```python
from build123d import *

# Parameters (mm, degrees)
F0_R     = 1.5
F1_DEPTH = 2.5


with BuildPart() as f1:
    # F0 (on Top) → F1 (new body)
    with BuildSketch(Plane.XY):
        Polygon((-24.927709, 2.481071), (7.530662, -30.014294), (11.431097, -31.130232), (23.566268, -40.223594), (34.787399, -29.015238), (46.00853, -17.806882), (36.928996, -5.66136), (35.817502, -1.759657), (3.359131, 30.735708), (-0.541304, 31.851646), (-12.676475, 40.945009), (-23.897606, 29.736653), (-35.118737, 18.528296), (-26.039203, 6.382775), align=None)
        with Locations((5.432613, -21.206046)):
            Circle(F0_R, mode=Mode.SUBTRACT)
        with Locations((23.566268, -33.655995)):
            Circle(F0_R, mode=Mode.SUBTRACT)
        with Locations((39.440935, -17.799401)):
            Circle(F0_R, mode=Mode.SUBTRACT)
        with Locations((27.01165, 0.348424)):
            Circle(F0_R, mode=Mode.SUBTRACT)
        with Locations((-16.121857, 0.372991)):
            Circle(F0_R, mode=Mode.SUBTRACT)
        with Locations((-28.551142, 18.520815)):
            Circle(F0_R, mode=Mode.SUBTRACT)
        with Locations((-12.676475, 34.37741)):
            Circle(F0_R, mode=Mode.SUBTRACT)
        with Locations((5.45718, 21.927461)):
            Circle(F0_R, mode=Mode.SUBTRACT)
    extrude(amount=F1_DEPTH)


solid = f1.part
```
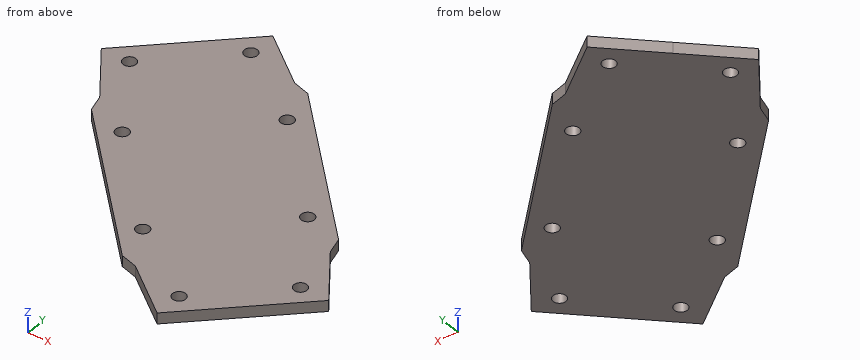
The listing builds one solid part. Answer for the finished solid, in the listing's coordinates (mm). Coordinates: 2 decimals unless noted, no trailing zeros. Write each loop counter-clockwise with the first axis right and the second up, starting at its lowest first coordinate (ties: lowest second). Pieces come first, ordered by that corner, then holes. Notation, with made-up numbers: (-36.5, -28.75) - (-18.5, -28.75) arc R22 cw to (-18.5, -22.75) - close; hole circle Ø8 at (27.5, 52). An arc over 180 degrees is marked (long way). One line per item, written item: value.
1) Each of these flat-tipped pins is pushed along its axis until it touches: pin 1 Ø6 at (x, y) = (10.5, -31) entering from +Z; pin 2 Ø1.5 at (x, z) = (31, 1.5) entering from +Y. Where does it stop, or does it pass through?
Geometry check:
pin 1: stops at z = 2.5
pin 2: stops at y = 3.81
2) Find section B-B (z = 1.8). Count the separate pieces of the cut face and the enclosed holes in it, and give its area (3 significant figures).
Geometry check:
separate pieces: 1
enclosed holes: 8
area: 3,070 mm2
3) Consider line 1 along Y through (x, z) = (28, 0.9); line 2 along X through (y, z) = (35, 1.8); line 3 along X through (y, z) = (-34, 1). Determine where each line is inside the solid, lowest interval first. Write a range as from..to.
Geometry check:
line 1: y = -35.79..-0.78, 1.48..6.07
line 2: x = -18.63..-14.04, -11.31..-4.74
line 3: x = 15.26..22.11, 25.03..29.8
4) Find section C-C (x = -29). Give the vertices of the cut face in (y, z), and give its area (3 significant figures).
Geometry check:
outline: (10.34, 0) - (17.09, 0) - (17.09, 2.5) - (10.34, 2.5) - close; (19.95, 0) - (24.64, 0) - (24.64, 2.5) - (19.95, 2.5) - close
area: 28.6 mm2
5) Find section D-D (y = -13). Give the vertices of the cut face in (x, z).
Geometry check:
outline: (-9.46, 0) - (42.42, 0) - (42.42, 2.5) - (-9.46, 2.5) - close
6) Find section A-A (x = 5.5). Give the vertices of the cut face in (y, z).
Geometry check:
outline: (-27.98, 0) - (-22.7, 0) - (-22.7, 2.5) - (-27.98, 2.5) - close; (-19.71, 0) - (20.43, 0) - (20.43, 2.5) - (-19.71, 2.5) - close; (23.43, 0) - (28.59, 0) - (28.59, 2.5) - (23.43, 2.5) - close
